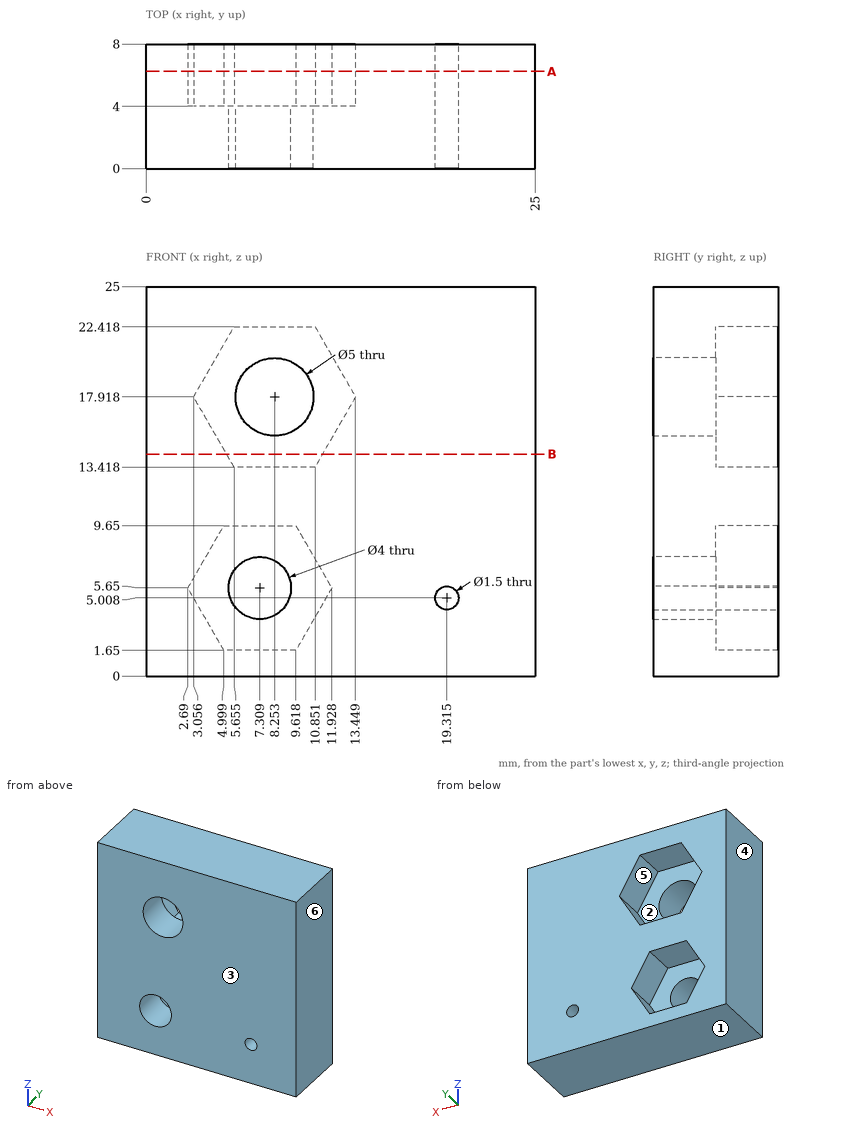
For this review, use the dimensioned drawing (mm, ordinates from the lowest corner) and the shaded views. A direction names the side the tool comes from. Coordinates: 2 decimals unless noted, no trailing zeros. Order: outer loops, then holes, each group sorted by start corner. A loop starts at its lowest first (then second) coordinate and runs counter-clockwise, first axis right, second up. Notation, with made-up numbers: (-15.75, 32) - (21.25, 32) arc R18 cw to (21.25, 43) - close; hole circle Ø5 at (-8, 60). An arc over 180 degrees is marked (long way). Answer as a JSON object with one key per item and string values. Group by question number.
1. For probe 1 along Z at (x, y) = (6.5, 0.75) (1 decimal); probe 2 along Z at (x, y) = (11, 5.25) (1 decimal); probe 3 along Y at (x, z) = (5.75, 17), list the stretches that pass through material, from the lowest coordinate up.
2. We need section A-A on y = 6.25. Give the number of separate pieces and of enclosed holes in the cut face, then the cut area to 3 significant figures.
3. We need section B-B on z = 14.25. State the section outline as (x, y) points, then the cut area to 3 significant figures.
4. For the marked faces 1 and 2, list the 3-axis set-ups (+Z, -Z, +X, -X, +Y, -Y) from which the entire face can be reached by the end or side of a thin tool; tool diameter is ignored.
5. The part is to be moulded in two halves that separate along X. For the marked faces 3, 4, 5 and 6, say which applies: pulls with the +X half, pulls with the -X half, needs draft (parallel to the pull), parting line crosses it, or undercut.
6. Clearance check with flat-ended pins moving along their axes: P1, Ø8, axis at x = 8.25, z = 17.92, coming from the +Y side; P2, Ø1.2, axis at x = 19.31, z = 5.01, coming from the -Y side. State where each tip first meets the part, or that it passes through.
Final values:
{
 "1": {"probe 1": "0 to 3.8, 7.5 to 16.1, 19.7 to 25", "probe 2": "0 to 4, 7.3 to 13.7, 22.2 to 25", "probe 3": "0 to 4"},
 "2": {"separate pieces": "1", "enclosed holes": "3", "area": "498 mm²"},
 "3": {"outline": "(0, 0) - (25, 0) - (25, 8) - (11.33, 8) - (11.33, 4) - (5.17, 4) - (5.17, 8) - (0, 8) - close", "area": "175 mm²"},
 "4": {"face 1": "-Z, +X, -X, +Y, -Y", "face 2": "+Y"},
 "5": {"face 3": "needs draft", "face 4": "pulls with the -X half", "face 5": "undercut", "face 6": "pulls with the +X half"},
 "6": {"P1": "y = 4", "P2": "through"}
}
